Could you check a few things on this model? Use its own coordinates, in mm. Give positions to 0.01 mm unless a question says otherwise; leave off trailing zeros.
(1) Will this pin go through, and if not, where does the flat tip stop? pin 1 (8 mm diameter, centred on x = 234.5, y = 12.76, fed in from +Z).
(2) If we mould it in two halves opening along X, with no side actions, what happens to faces 1 (the cylindrical face through (113.305, 14.223, 1.034)), 2 (the flat face through (138.9, 7.6, 0)), 3 (the cylindrical face through (3.77, 3.97, 1.03))? For each: released by +X, released by -X, zero draft, split by the parting line, or undercut.
(3) If I drill on probe 1 along Y at (x, z) = (242.5, 0.5); probe 2 along Y at (x, z) = (219, 0.4); probe 3 along Y at (x, z) = (78.5, 0.6), over which ranges is the centre line in solid material (lowest first)?
(4) Imagine slicing it at A-A, the plane z = 1.35. State how many separate pieces and enclosed holes the cut face has, then the cut area to 3 significant figures.
Autodesk Inventor part; units mm, degrees
ref_plane "YZ Plane" through (0, 0, 0) normal (1, 0, 0) x (0, 1, 0)
ref_plane "XZ Plane" through (0, 0, 0) normal (0, 1, 0) x (-1, 0, 0)
ref_plane "XY Plane" through (0, 0, 0) normal (0, 0, 1) x (1, 0, 0)
sketch "Sketch1" plane through (0, 0, 0) normal (0, 0, 1) x (1, 0, 0)
  line L0 (0, 0) -> (281.7812, 0)
  line L1 (281.7812, 0) -> (281.7812, 26.57)
  line L2 (281.7812, 26.57) -> (0, 26.57)
  line L3 (0, 26.57) -> (0, 0)
  dimension "d0" = 281.7812
  dimension "d1" = 26.57
extrude "Extrusion1" add sketch "Sketch1" along normal blind 2.04
sketch "Sketch2" plane through (0, 0, 2.04) normal (0, 0, 1) x (1, 0, 0)
  line L0 (0, 26.57) -> (0, 0)
  line L1 (0, 0) -> (0, 12.7584)
  line L2 (0, 12.7584) -> (14.275, 12.7584)
  line L3 (0, 12.7584) -> (14.275, 12.7584) construction
  circle A0 centre (14.275, 12.7584) radius 4.875
  line L4 (14.275, 12.7584) -> (16.815, 12.7584)
  circle A1 centre (30.005, 12.7584) radius 4.875
  circle A2 centre (45.735, 12.7584) radius 4.875
  circle A3 centre (61.465, 12.7584) radius 4.875
  circle A4 centre (77.195, 12.7584) radius 4.875
  circle A5 centre (92.925, 12.7584) radius 4.875
  circle A6 centre (108.655, 12.7584) radius 4.875
  circle A7 centre (124.385, 12.7584) radius 4.875
  circle A8 centre (140.115, 12.7584) radius 4.875
  circle A9 centre (155.845, 12.7584) radius 4.875
  circle A10 centre (171.575, 12.7584) radius 4.875
  circle A11 centre (187.305, 12.7584) radius 4.875
  circle A12 centre (203.035, 12.7584) radius 4.875
  circle A13 centre (218.765, 12.7584) radius 4.875
  circle A14 centre (234.495, 12.7584) radius 4.875
  circle A15 centre (250.225, 12.7584) radius 4.875
  circle A16 centre (265.955, 12.7584) radius 4.875
  dimension "d4" = 12.7584
  dimension "d5" = 14.275
  dimension "d6" = 0
  dimension "d7" = 9.75
  dimension "d8" = 2.54
  dimension "d13" = 15.73
extrude "Extrusion2" cut sketch "Sketch2" against normal blind 2.04
fillet "Fillet1" radius 13.208 4 edges at (0, 26.57, 1.02) (0, 0, 1.02) (281.7812, 26.57, 1.02) (281.7812, 0, 1.02)
sketch "Sketch3" plane through (0, 0, 2.04) normal (0, 0, 1) x (1, 0, 0)
  line L0 (13.208, 0) -> (268.5733, 0)
  line L1 (0, 13.362) -> (0, 13.208)
  circle A0 centre (14.275, 12.7584) radius 4.875
  line L2 (14.275, 7.8834) -> (14.275, 17.6334)
  line L3 (9.4, 12.7584) -> (19.15, 12.7584)
  line L4 (14.275, 12.7584) -> (14.275, 20.6234)
  line L5 (268.5733, 26.57) -> (13.208, 26.57)
  line L6 (10.8279, 9.3113) -> (17.7221, 16.2056)
  line L7 (14.275, 7.8834) -> (14.275, 17.6334)
  line L8 (17.7221, 9.3113) -> (10.8279, 16.2056)
  line L9 (19.15, 12.7584) -> (9.4, 12.7584)
  line L10 (17.7221, 16.2056) -> (10.8279, 9.3113)
  line L11 (14.275, 17.6334) -> (14.275, 7.8834)
  line L12 (10.8279, 16.2056) -> (17.7221, 9.3113)
  point P0 (0, 0)
  point P1 (8.7136, 18.3198)
  point P2 (6.41, 12.7584)
  point P3 (8.7136, 7.197)
  point P4 (14.275, 4.8934)
  point P5 (19.8364, 7.197)
  point P6 (22.14, 12.7584)
  point P7 (19.8364, 18.3198)
  dimension "d30" = 360
  dimension "d39" = 7.865
hole "Hole1" at (14.275, 20.6234, 2.04) at (8.7136, 18.3198, 2.04) at (6.41, 12.7584, 2.04) at (8.7136, 7.197, 2.04) at (14.275, 4.8934, 2.04) at (19.8364, 7.197, 2.04) at (22.14, 12.7584, 2.04) at (19.8364, 18.3198, 2.04) direction (0, 0, -1) diameter 3.5 end through all
pattern_linear "Rectangular Pattern1" count 5 spacing 62.92 along (1, 0, 0) of "Hole1"
sketch "Sketch4" plane through (0, 0, 2.04) normal (0, 0, 1) x (1, 0, 0)
  line L0 (45.5847, 12.7584) -> (45.5847, 20.6234)
  circle A0 centre (30.005, 12.7584) radius 4.875
  line L1 (30.005, 12.7584) -> (35.5959, 12.7584)
  line L2 (30.005, 12.7584) -> (35.5959, 12.7584) construction
  line L3 (30.005, 12.7584) -> (45.5847, 12.7584)
  point P0 (0, 0)
  point P1 (37.7197, 12.7584)
  point P2 (45.5847, 4.8934)
  point P3 (53.4497, 12.7584)
  point P4 (116.3697, 12.7584)
  point P5 (108.5047, 4.8934)
  point P6 (100.6397, 12.7584)
  point P7 (108.5047, 20.6234)
  point P8 (179.2897, 12.7584)
  point P9 (171.4247, 4.8934)
  point P10 (163.5597, 12.7584)
  point P11 (171.4247, 20.6234)
  point P12 (242.2097, 12.7584)
  point P13 (234.3447, 4.8934)
  point P14 (226.4797, 12.7584)
  point P15 (234.3447, 20.6234)
  dimension "d43" = 7.865
  dimension "d46" = 360
  dimension "d48" = 0
  dimension "d49" = 15.5797
  dimension "d52" = 62.92
hole "Hole2" at (45.5847, 4.8934, 2.04) at (53.4497, 12.7584, 2.04) at (45.5847, 20.6234, 2.04) at (37.7197, 12.7584, 2.04) at (100.6397, 12.7584, 2.04) at (108.5047, 4.8934, 2.04) at (116.3697, 12.7584, 2.04) at (108.5047, 20.6234, 2.04) at (171.4247, 20.6234, 2.04) at (179.2897, 12.7584, 2.04) at (171.4247, 4.8934, 2.04) at (163.5597, 12.7584, 2.04) at (234.3447, 4.8934, 2.04) at (226.4797, 12.7584, 2.04) at (242.2097, 12.7584, 2.04) at (234.3447, 20.6234, 2.04) direction (0, 0, -1) diameter 3.5 end through all
properties part number "max length flat tetrix part"
Answer block:
1. pin 1: passes through
2. face 1: undercut
2. face 2: zero draft
2. face 3: released by -X
3. probe 1: y = 0 to 11.03, 14.48 to 26.57
3. probe 2: y = 0 to 7.89, 17.63 to 26.57
3. probe 3: y = 0 to 3.73, 6.06 to 8.06, 17.46 to 19.46, 21.79 to 26.57
4. separate pieces: 1
4. enclosed holes: 73
4. area: 5,530 mm2
